```python
from build123d import *

# Parameters (mm, degrees)
SKETCH_1_R            = 10
SKETCH_1_R_2          = 5
EXTRUDE_2_DEPTH       = 10
SKETCH_3_R            = 2.5
EXTRUDE_4_DEPTH       = 10
EXTRUDE_1_OUTLINE_W   = 50
EXTRUDE_1_OUTLINE_H   = 40
EXTRUDE_1_OUTLINE_W_2 = 40
EXTRUDE_1_OUTLINE_H_2 = 30
EXTRUDE_1_DEPTH       = 20
EXTRUDE_1_2_OUTLINE_W = 40
EXTRUDE_1_2_OUTLINE_H = 30
EXTRUDE_1_2_DEPTH     = 5
EXTRUDE_START         = 15
EXTRUDE_1_3_OUTLINE_W = 40
EXTRUDE_1_3_OUTLINE_H = 30
EXTRUDE_1_3_DEPTH     = 5
EXTRUDE_2_2_DEPTH     = 5
SKETCH_15_R           = 2.5
CUT_EXTRUDE_3_DEPTH   = 15
SKETCH_20_W           = 16
SKETCH_20_H           = 11
CUT_EXTRUDE_7_DEPTH   = 10


# Read off the part's stored shape, not the designer's step: 拉伸-薄壁1
with BuildPart() as part:
    # 草图1 → Extrude 2 (new body)
    # profile 1 of 7: a face of its own
    with BuildSketch(Plane(origin=(0, 0, 0), x_dir=(1, 0, 0), z_dir=(0, 1, 0))):
        with BuildLine():
            Line((70, 0), (40, 0))
            Line((40, 0), (40, -30))
            Line((40, -30), (40, -60))
            Line((40, -60), (70, -60))
            ThreePointArc((70, -60), (62.928932188, -42.928932188), (80, -50))
            Line((80, -50), (80, -10))
            ThreePointArc((80, -10), (62.928932188, -17.071067812), (70, 0))
        make_face()
    # profile 2 of 7: a face of its own
    with BuildSketch(Plane(origin=(0, 0, 0), x_dir=(1, 0, 0), z_dir=(0, 1, 0))):
        with BuildLine():
            Line((40, -30), (40, 0))
            Line((40, 0), (10, 0))
            ThreePointArc((10, 0), (17.071067812, -2.928932188), (20, -10))
            ThreePointArc((20, -10), (10, -20), (0, -10))
            Line((0, -10), (0, -30))
            Line((0, -30), (40, -30))
        make_face()
    # profile 3 of 7: a face of its own
    with BuildSketch(Plane(origin=(0, 0, 0), x_dir=(1, 0, 0), z_dir=(0, 1, 0))):
        with BuildLine():
            Line((40, -60), (40, -30))
            Line((40, -30), (0, -30))
            Line((0, -30), (0, -50))
            ThreePointArc((0, -50), (10, -40), (20, -50))
            ThreePointArc((20, -50), (17.071067812, -57.071067812), (10, -60))
            Line((10, -60), (40, -60))
        make_face()
    # profile 4 of 7: a face of its own
    with BuildSketch(Plane(origin=(0, 0, 0), x_dir=(1, 0, 0), z_dir=(0, 1, 0))):
        with Locations((10, -50)):
            Circle(SKETCH_1_R)
        with Locations(Location((10, -50, 0), (0, 0, 270))):
            Circle(SKETCH_1_R_2, mode=Mode.SUBTRACT)
    # profile 5 of 7: a face of its own
    with BuildSketch(Plane(origin=(0, 0, 0), x_dir=(1, 0, 0), z_dir=(0, 1, 0))):
        with Locations((70, -50)):
            Circle(SKETCH_1_R)
        with Locations(Location((70, -50, 0), (0, 0, 270))):
            Circle(SKETCH_1_R_2, mode=Mode.SUBTRACT)
    # profile 6 of 7: a face of its own
    with BuildSketch(Plane(origin=(0, 0, 0), x_dir=(1, 0, 0), z_dir=(0, 1, 0))):
        with Locations((70, -10)):
            Circle(SKETCH_1_R)
        with Locations(Location((70, -10, 0), (0, 0, 270))):
            Circle(SKETCH_1_R_2, mode=Mode.SUBTRACT)
    # profile 7 of 7: a face of its own
    with BuildSketch(Plane(origin=(0, 0, 0), x_dir=(1, 0, 0), z_dir=(0, 1, 0))):
        with Locations((10, -10)):
            Circle(SKETCH_1_R)
        with Locations(Location((10, -10, 0), (0, 0, 270))):
            Circle(SKETCH_1_R_2, mode=Mode.SUBTRACT)
    extrude(amount=EXTRUDE_2_DEPTH)

    # 草图3 → 凸台-拉伸4 (add)
    with BuildSketch(Plane.XY.offset(60)):
        with BuildLine():
            Line((25, 16), (25, 10))
            Line((25, 10), (35, 10))
            Line((35, 10), (35, 16))
            ThreePointArc((35, 16), (30, 21), (25, 16))
        make_face()
        with Locations((30, 16)):
            Circle(SKETCH_3_R, mode=Mode.SUBTRACT)
    extrude(amount=-EXTRUDE_4_DEPTH)

    # 拉伸-薄壁1 outline → 拉伸-薄壁1 (add)
    with BuildSketch(Plane(origin=(0, 10, 0), x_dir=(1, 0, 0), z_dir=(0, 1, 0))):
        with Locations((40, -30)):
            Rectangle(EXTRUDE_1_OUTLINE_W, EXTRUDE_1_OUTLINE_H)
        with Locations((40, -30)):
            Rectangle(EXTRUDE_1_OUTLINE_W_2, EXTRUDE_1_OUTLINE_H_2, mode=Mode.SUBTRACT)
    extrude(amount=EXTRUDE_1_DEPTH)

    # Extrude 1 2 outline → Extrude 1 2 (add)
    with BuildSketch(Plane(origin=(0, 10, 0), x_dir=(1, 0, 0), z_dir=(0, 1, 0))):
        with Locations((40, -30)):
            Rectangle(EXTRUDE_1_2_OUTLINE_W, EXTRUDE_1_2_OUTLINE_H)
    extrude(amount=EXTRUDE_1_2_DEPTH)

    # Extrude 1 3 outline → Extrude 1 3 (add)
    with BuildSketch(Plane(origin=(0, 10, 0), x_dir=(1, 0, 0), z_dir=(0, 1, 0)).offset(EXTRUDE_START)):
        with Locations((40, -30)):
            Rectangle(EXTRUDE_1_3_OUTLINE_W, EXTRUDE_1_3_OUTLINE_H)
    extrude(amount=EXTRUDE_1_3_DEPTH)

    # 草图14 → Extrude 2 2 (add)
    with BuildSketch(Plane(origin=(0, 30, 0), x_dir=(1, 0, 0), z_dir=(0, 1, 0))):
        Polygon((30, -37.5), (30, -22.5), (40, -22.5), (50, -22.5), (50, -37.5), (40, -37.5), align=None)
        Polygon((32, -35.5), (32, -24.5), (40, -24.5), (48, -24.5), (48, -35.5), (40, -35.5), align=None, mode=Mode.SUBTRACT)
    extrude(amount=EXTRUDE_2_2_DEPTH)

    # 草图15 → 切除-拉伸3 (cut)
    with BuildSketch(Plane.XY.offset(60)):
        with Locations((30, 16)):
            Circle(SKETCH_15_R)
    extrude(amount=-CUT_EXTRUDE_3_DEPTH, mode=Mode.SUBTRACT)

    # 草图20 → 切除-拉伸7 (cut)
    with BuildSketch(Plane(origin=(0, 30, 0), x_dir=(1, 0, 0), z_dir=(0, 1, 0))):
        with Locations((40, -30)):
            Rectangle(SKETCH_20_W, SKETCH_20_H)
    extrude(amount=-CUT_EXTRUDE_7_DEPTH, mode=Mode.SUBTRACT)


solid = part.part
```
Verification items for the finished model (mm, model axes). A direction names the side the tool comes from. Give positions to 0.01 mm unless a question says otherwise; leave off trailing zeros. Write each loop counter-clockwise with the first axis right and the second up, starting at its lowest first coordinate (ties: lowest second). Pieces come first, ordered by that corner, then holes. Notation, with made-up numbers: M -18,-30 L 7,-30 A26 ccw 7,-4 Z; hole C -3.5,12.5 d6. An arc over 180 degrees is marked long. One line per question, with ' | ' between items.
1) Thickness scan on line 1 along Z through (x, y) = (70, 7); line 2 along X through (y, z) = (6.75, 50); line 3 along X through (y, z) = (22.5, 40.5). Record the ranges inside material, lowest first. Write a range as [from, to].
Result:
line 1: z = [0, 5], [15, 45], [55, 60] | line 2: x = [0, 5], [15, 65], [75, 80] | line 3: x = [15, 20], [60, 65]
2) Mould release check, pull along X, two halves, no side actions. Record for faces 1 (the cylindrical face through (76.99, 4.93, 57.15)), 2 (the flat face through (39.4, 10, 9.6)), 3 (the cylindrical face through (28, 14.5, 52.6)): released by +X, released by -X, zero draft, split by the parting line, or undercut.
Result:
face 1: released by +X | face 2: zero draft | face 3: undercut
3) Section check A-A on x = 66. Enter the section's corners in (y, z).
Result:
outline: M 0,0 L 10,0 L 10,7 L 0,7 Z; M 0,13 L 10,13 L 10,47 L 0,47 Z; M 0,53 L 10,53 L 10,60 L 0,60 Z
4) Section check B-B on y = 7. Enter the section's corners in (x, z).
Result:
outline: M 0,10 A10 ccw 10,0 L 70,0 A10 ccw 80,10 L 80,50 A10 ccw 70,60 L 10,60 A10 ccw 0,50 Z; hole C 10,10 d10; hole C 10,50 d10; hole C 70,10 d10; hole C 70,50 d10
5) Gauge pin test, flat ends, axial feed: pin 1 Ø4 at (x, y) = (42, 33) entering from +Z; pin 2 Ø5 at (y, z) = (20, 33.5) entering from +X; pin 3 Ø3 at (y, z) = (21.5, 28.5) entering from -X. Record the tip position at first contact, or that the pin passes through.
Result:
pin 1: stops at z = 37.5 | pin 2: stops at x = 65 | pin 3: stops at x = 15
6) Set-up check for faces 4 (the flat face through (48, 30, 30)), 5 (the flat face through (40, 32, 37.5)), 6 (the flat face through (40, 20, 10)), 7 (the flat face through (65, 20, 30)): record each of +Z, -Z, +X, -X, +Y, -Y from which the full face is reachable in a straight line by a thin tool's end or side.
Result:
face 4: +Y | face 5: +Z, +X, -X, +Y | face 6: -Z, +X, -X, +Y | face 7: +Z, -Z, +X, +Y
7) Section check C-C on z = 53.5. Enter the section's corners in (x, y).
Result:
outline: M 0.63,0 L 6.43,0 L 6.43,10 L 0.63,10 Z; M 13.57,0 L 66.43,0 L 66.43,10 L 35,10 L 35,16 A5 ccw 25,16 L 25,10 L 13.57,10 Z; M 73.57,0 L 79.37,0 L 79.37,10 L 73.57,10 Z; hole C 30,16 d5
8) Section check D-D on x = 43.5. Enter the section's corners in (y, z), plus the area to 4 significant figures.
Result:
outline: M 0,0 L 10,0 L 10,10 L 30,10 L 30,22.5 L 35,22.5 L 35,24.5 L 25,24.5 L 25,15 L 15,15 L 15,45 L 25,45 L 25,35.5 L 35,35.5 L 35,37.5 L 30,37.5 L 30,50 L 10,50 L 10,60 L 0,60 Z | area: 1,065 mm2
